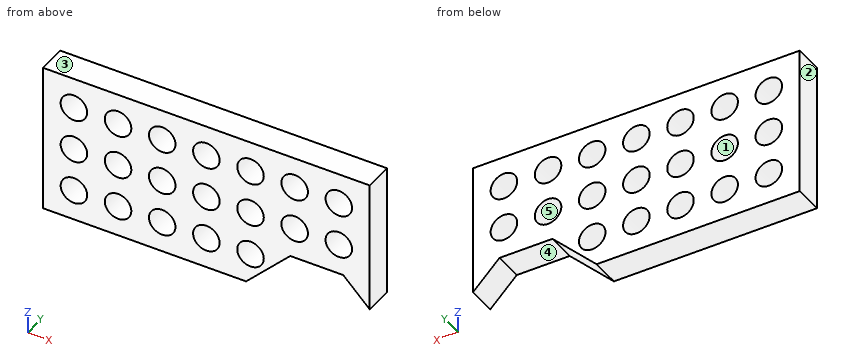
```python
from build123d import *

# Parameters (mm, degrees)
SKETCH1_R           = 1.5025
BOSS_EXTRUDE1_DEPTH = 3.25


with BuildPart() as part:
    # Sketch1 → Boss-Extrude1 (new body)
    with BuildSketch(Plane(origin=(0, 0, 0), x_dir=(1, 0, 0), z_dir=(0, 1, 0))):
        Polygon((-18.5, 8.5), (4.5, 8.5), (9.5, 3.5), (15.5, 3.5), (18.5, 6.5), (18.5, -8.5), (-18.5, -8.5), align=None)
        with Locations((-15, -5)):
            Circle(SKETCH1_R, mode=Mode.SUBTRACT)
        with Locations((-10, -5)):
            Circle(SKETCH1_R, mode=Mode.SUBTRACT)
        with Locations((-5, -5)):
            Circle(SKETCH1_R, mode=Mode.SUBTRACT)
        with Locations((0, -5)):
            Circle(SKETCH1_R, mode=Mode.SUBTRACT)
        with Locations((5, -5)):
            Circle(SKETCH1_R, mode=Mode.SUBTRACT)
        with Locations((10, -5)):
            Circle(SKETCH1_R, mode=Mode.SUBTRACT)
        with Locations((15, -5)):
            Circle(SKETCH1_R, mode=Mode.SUBTRACT)
        with Locations((-10, 0)):
            Circle(SKETCH1_R, mode=Mode.SUBTRACT)
        with Locations((-5, 0)):
            Circle(SKETCH1_R, mode=Mode.SUBTRACT)
        Circle(SKETCH1_R, mode=Mode.SUBTRACT)
        with Locations((5, 0)):
            Circle(SKETCH1_R, mode=Mode.SUBTRACT)
        with Locations((10, 0)):
            Circle(SKETCH1_R, mode=Mode.SUBTRACT)
        with Locations((15, 0)):
            Circle(SKETCH1_R, mode=Mode.SUBTRACT)
        with Locations((-10, 5)):
            Circle(SKETCH1_R, mode=Mode.SUBTRACT)
        with Locations((-5, 5)):
            Circle(SKETCH1_R, mode=Mode.SUBTRACT)
        with Locations((0, 5)):
            Circle(SKETCH1_R, mode=Mode.SUBTRACT)
        with Locations((5, 5)):
            Circle(SKETCH1_R, mode=Mode.SUBTRACT)
        with Locations((-15, 0)):
            Circle(SKETCH1_R, mode=Mode.SUBTRACT)
        with Locations((-15, 5)):
            Circle(SKETCH1_R, mode=Mode.SUBTRACT)
    extrude(amount=BOSS_EXTRUDE1_DEPTH)


solid = part.part
```
Model file for the job. Use its own axes, mm. Face numbers are marked on the shaded views. A direction names the side the tool comes from. Coordinates: 2 decimals unless noted, no trailing zeros. Loops run counter-clockwise (first coordinate to the right, second up) from the corner with the lowest first, then second, coordinate; pieces in that order, holes last. Notation, with made-up numbers: (25, 57.25) - (46, 57.25) arc R13 ccw to (46, 65.25) - close; hole circle Ø11 at (55, -26.5). An arc over 180 degrees is marked (long way). Write item = value, one per line. Start each with the question number.
Item 1: Wall check: probe 1 along Z at (x, y) = (0, 1.4); probe 2 along Z at (x, y) = (15, 1.6); probe 3 along Z at (x, y) = (5, 1). Give the ranges that are in metal, low to high. Write a range as [from, to].
Item 2: Pull direction X, two halves, no side cores. Call the marked faces 1, 2 and 3: +X half, -X half, draft (parallel to the pull), parting line (faces both ways), or undercut.
Item 3: Saw through at B-B, the plane z = -5. List the corners of the cut face in (x, y).
Item 4: Saw through at D-D, the plane y = 2.75. State how many separate pieces and enclosed holes the cut face has, then the cut area to 3 significant figures.
Item 5: Saw through at C-C, the plane x = 15. List the corners of the cut face in (y, z), then the cut area to 3 significant figures.
Item 6: 3-axis set-ups, long thin cutter, end or side, ignore diameter. For the marked faces 4 and 5: which of +Z, -Z, +X, -X, +Y, -Y reach the whole face in a straight line?
Item 7: Drop flat-ended pins along their axis: pin 1 Ø1.6 at (x, y) = (13.5, 1.5) entering from -Z; pin 2 Ø3.5 at (x, z) = (5, 0) entering from -Y; pin 3 Ø1.5 at (x, y) = (9.5, 1.5) entering from -Z. Give the stop position or say it passes through.
Item 8: Saw through at A-A, the plane x = 5. List the corners of the cut face in (y, z), then the cut area to 3 significant figures.
Answers:
q1.probe_1 = [-8.5, -6.5], [-3.5, -1.5], [1.5, 3.5], [6.5, 8.5]
q1.probe_2 = [-3.5, -1.5], [1.5, 3.5], [6.5, 8.5]
q1.probe_3 = [-8, -6.5], [-3.5, -1.5], [1.5, 3.5], [6.5, 8.5]
q2.face_1 = undercut
q2.face_2 = -X half
q2.face_3 = draft
q3.outline = (-18.5, 0) - (-16.5, 0) - (-16.5, 3.25) - (-18.5, 3.25) - close; (-13.5, 0) - (-11.5, 0) - (-11.5, 3.25) - (-13.5, 3.25) - close; (-8.5, 0) - (-6.5, 0) - (-6.5, 3.25) - (-8.5, 3.25) - close; (-3.5, 0) - (-1.5, 0) - (-1.5, 3.25) - (-3.5, 3.25) - close; (1.5, 0) - (3.5, 0) - (3.5, 3.25) - (1.5, 3.25) - close; (6.5, 0) - (8, 0) - (8, 3.25) - (6.5, 3.25) - close; (17, 0) - (18.5, 0) - (18.5, 3.25) - (17, 3.25) - close
q4.separate_pieces = 1
q4.enclosed_holes = 19
q4.area = 441 mm2
q5.outline = (0, -3.5) - (3.25, -3.5) - (3.25, -1.5) - (0, -1.5) - close; (0, 1.5) - (3.25, 1.5) - (3.25, 3.5) - (0, 3.5) - close; (0, 6.5) - (3.25, 6.5) - (3.25, 8.5) - (0, 8.5) - close
q5.area = 19.5 mm2
q6.face_4 = -Z, +Y, -Y
q6.face_5 = +Y, -Y
q7.pin_1 = -3.5
q7.pin_2 = 0
q7.pin_3 = -4.25
q8.outline = (0, -8) - (3.25, -8) - (3.25, -6.5) - (0, -6.5) - close; (0, -3.5) - (3.25, -3.5) - (3.25, -1.5) - (0, -1.5) - close; (0, 1.5) - (3.25, 1.5) - (3.25, 3.5) - (0, 3.5) - close; (0, 6.5) - (3.25, 6.5) - (3.25, 8.5) - (0, 8.5) - close
q8.area = 24.3 mm2
